Work out the finished part from the listing and answer in its coordinate system (mm). A direction names the side the tool comes from. Give positions to 0.01 mm unless a question says otherwise; leave off trailing zeros. Write each loop counter-clockwise with the first axis right and the second up, starting at its lowest first coordinate (ties: lowest second). Pieces come first, ordered by that corner, then holes. Notation, with made-up numbers: (88, -25) -> (139, -25) arc R26 ccw to (139, 5) -> close; hole circle Ø9 at (2, -28). An arc over 180 degrees is marked (long way). Use a Markdown table: item, result. Add a question column.
Q1. For faces 4 (the face through (0, 1, 0)), 5 (the face through (986, 3, -1)), determine the directions among +Z, -Z, +X, -X, +Y, -Y from which every point of the face is accessible in a straight line to the end or side of a thin tool.
Q2. Section B-B, the plane x = 1612.5 is taken. Give the vertices of the cut face in (y, z), plus the area to 3 significant figures.
Q3. Each of these flat-tipped pins is pushed along its axis until it touches: pin 1 Ø19 at (x, z) = (200, 50) entering from +Y; pin 2 Ø2 at (x, z) = (526, 0) entering from +Y. Where does it stop, or does it pass through?
Q4. Consider line 1 (Z direction, x = 200, y = 1.85); line 2 (Z direction, x = 669, y = 31); line 3 (Y direction, x = 1451.5, z = -88). Determine where each line is inside the solid, lowest interval first.
Q5. Section C-C, the plane z = -15.5 is taken. Give the vertices of the cut face in (x, y), plus the area to 3 significant figures.
Q6. For a pull along Z with two mould halves and no side action, classify faces 1 (the face through (986, 41, 100)), 2 (the face through (986, 39, -100)), 3 (the face through (986, 39, 97)) as pulls with the +Z half, pulls with the -Z half, needs draft (parallel to the pull), parting line crosses it, or undercut.
Q7. Section A-A, the plane y = 22.5 is taken. Give the vertices of the cut face in (x, z).
from build123d import *

# Parameters (mm, degrees)
F1_DEPTH = 2000
F2_R     = 10.626001
F3_DEPTH = 25
F4_R     = 10.626001
F5_DEPTH = 25


with BuildPart() as f1:
    # F0 (on Right) → F1 (new body)
    with BuildSketch(Plane.YZ):
        Polygon((0, 100), (0, 0), (0, -100), (80, -100), (80, -73.984891), (77, -73.984891), (77, -97), (3, -97), (3, 0), (3, 97), (77, 97), (77, 73.984891), (80, 73.984891), (80, 100), align=None)
    extrude(amount=F1_DEPTH)

    # F2 (on face) → F3 (cut)
    with BuildSketch(Plane.XZ):
        with Locations((200, 50)):
            Circle(F2_R)
        with Locations((200, -50)):
            Circle(F2_R)
        with Locations((350, 50)):
            Circle(F2_R)
        with Locations((350, -50)):
            Circle(F2_R)
    extrude(amount=-F3_DEPTH, mode=Mode.SUBTRACT)

    # F4 (on face) → F5 (cut)
    with BuildSketch(Plane.XZ):
        with Locations((1650, 50)):
            Circle(F4_R)
        with Locations((1650, -50)):
            Circle(F4_R)
        with Locations((1800, 50)):
            Circle(F4_R)
        with Locations((1800, -50)):
            Circle(F4_R)
    extrude(amount=-F5_DEPTH, mode=Mode.SUBTRACT)


solid = f1.part
Result set:
| question | item | result |
|---|---|---|
| 1 | face 4 | +Z, -Z, -X, +Y, -Y |
| 1 | face 5 | +X, -X |
| 2 | outline | (0, -100) -> (80, -100) -> (80, -73.98) -> (77, -73.98) -> (77, -97) -> (3, -97) -> (3, 97) -> (77, 97) -> (77, 73.98) -> (80, 73.98) -> (80, 100) -> (0, 100) -> close |
| 2 | area | 1,200 mm2 |
| 3 | pin 1 | passes through |
| 3 | pin 2 | stops at y = 3 |
| 4 | line 1 | z = -100 to -60.63, -39.37 to 39.37, 60.63 to 100 |
| 4 | line 2 | z = -100 to -97, 97 to 100 |
| 4 | line 3 | y = 0 to 3, 77 to 80 |
| 5 | outline | (0, 0) -> (2000, 0) -> (2000, 3) -> (0, 3) -> close |
| 5 | area | 6,000 mm2 |
| 6 | face 1 | pulls with the +Z half |
| 6 | face 2 | pulls with the -Z half |
| 6 | face 3 | undercut |
| 7 | outline | (0, -100) -> (2000, -100) -> (2000, -97) -> (0, -97) -> close; (0, 97) -> (2000, 97) -> (2000, 100) -> (0, 100) -> close |
